Here's the drawing with two shaded views (mm, measured from the low corner). I have some questions. Round coordinates to 2 decimals unless told otherwise and drop trailing zeros. Loops run counter-clockwise (first coordinate to the right, second up) from the corner with the lowest first, then second, coordinate; pieces in that order, holes last. Notation, with made-up numbers: (9.5, 68.5) -> (62.5, 68.5) arc R16 ccw to (62.5, 78.5) -> close; hole circle Ø8 at (32, 87). An arc over 180 degrees is marked (long way). Write item = value, one per line.
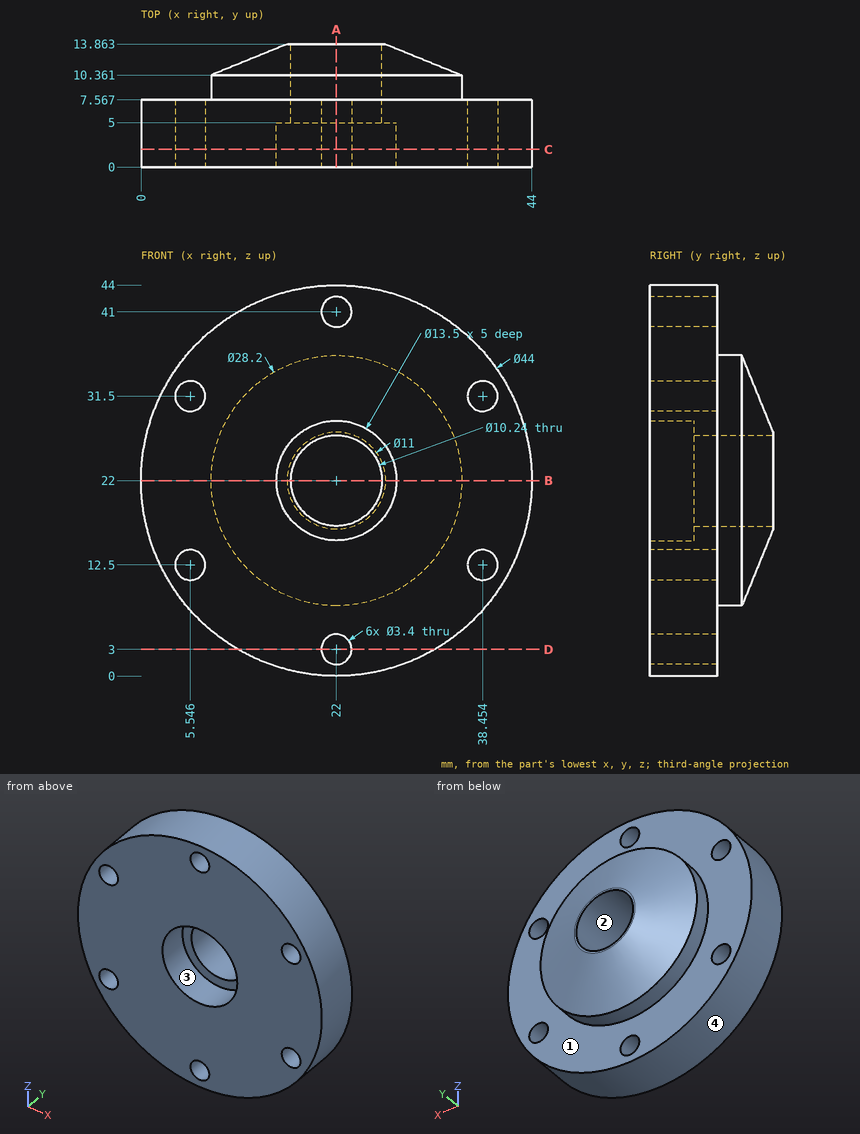
1. We'd pull the mould along X, two halves only. Please class the marked faces 1, 2, 3 and 4: released by +X, released by -X, zero draft, split by the parting line, or undercut.
Entries:
face_1 = zero draft
face_2 = undercut
face_3 = undercut
face_4 = split by the parting line
2. I need wall thicknesses on line 1 (X direction, y = 3.75, z = 31.5) (1 decimal); line 2 (Z direction, x = 4.5, y = 4) (1 decimal); line 3 (Y direction, x = 8.5, z = 9). Which ranges of each line are inside material? Lowest first, please. Write a range as [from, to].
Entries:
line_1 = [2.2, 3.8], [7.2, 36.8], [40.2, 41.8]
line_2 = [8.7, 11.2], [13.8, 30.2], [32.8, 35.3]
line_3 = [0, 7.57]
3. Suppose I cut it at D-D, the plane z = 3. List the corners of the cut face in (x, y) for me, and give its area (3 significant figures).
Entries:
outline = (10.91, 0) -> (20.3, 0) -> (20.3, 7.57) -> (10.91, 7.57) -> close; (23.7, 0) -> (33.09, 0) -> (33.09, 7.57) -> (23.7, 7.57) -> close
area = 142 mm²
4. Suppose I cut it at B-B, the plane z = 22. List the corners of the cut face in (x, y) for me.
Entries:
outline = (0, 0) -> (15.25, 0) -> (15.25, 5) -> (16.88, 5) -> (16.88, 13.86) -> (16.5, 13.86) -> (7.9, 10.36) -> (7.9, 7.57) -> (0, 7.57) -> close; (27.12, 5) -> (28.75, 5) -> (28.75, 0) -> (44, 0) -> (44, 7.57) -> (36.1, 7.57) -> (36.1, 10.36) -> (27.5, 13.86) -> (27.12, 13.86) -> close
5. Suppose I cut it at A-A, the plane x = 22. List the corners of the cut face in (y, z) for me, and give its area (3 significant figures).
Entries:
outline = (0, 0) -> (7.57, 0) -> (7.57, 1.3) -> (0, 1.3) -> close; (0, 4.7) -> (7.57, 4.7) -> (7.57, 7.9) -> (10.36, 7.9) -> (13.86, 16.5) -> (13.86, 16.88) -> (5, 16.88) -> (5, 15.25) -> (0, 15.25) -> close; (0, 28.75) -> (5, 28.75) -> (5, 27.12) -> (13.86, 27.12) -> (13.86, 27.5) -> (10.36, 36.1) -> (7.57, 36.1) -> (7.57, 39.3) -> (0, 39.3) -> close; (0, 42.7) -> (7.57, 42.7) -> (7.57, 44) -> (0, 44) -> close
area = 271 mm²
6. I'm going to push flat-ended pins straight in: pin 1 (8 mm diameter, centred on y = 9, z = 36.5, fed in from -X) (1 decimal); pin 2 (2 mm diameter, centred on x = 6.5, z = 23.5, fed in from +Y); pin 3 (1 mm diameter, centred on y = 2, z = 29.5, fed in from +X). Where does each tip first touch, or does it pass through?
Entries:
pin_1 = 2.8
pin_2 = 7.57
pin_3 = 42.86
7. Suppose I cut it at C-C, the plane y = 2. Count the separate pieces of the cut face and the enclosed holes in it, and give its area (3 significant figures).
Entries:
separate_pieces = 1
enclosed_holes = 7
area = 1,320 mm²
